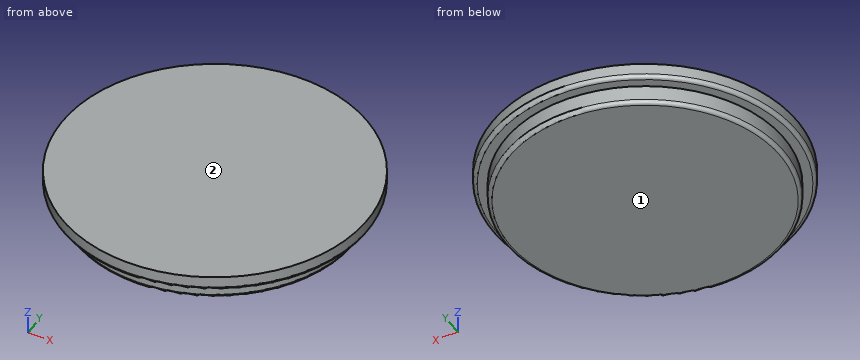
```python
from build123d import *

# Parameters (mm, degrees)
F0_R     = 18.75
F1_DEPTH = 2.5
F2_R     = 0.5
F3_R     = 20.5
F4_DEPTH = 2
F5_R     = 0.5


with BuildPart() as f1:
    # F0 (on Top) → F1 (new body)
    with BuildSketch(Plane.XY):
        Circle(F0_R)
    extrude(amount=F1_DEPTH)

    # F2
    f2_edges = [f1.edges().sort_by_distance(p)[0] for p in [
        (-18.75, 0, 0),
    ]]
    fillet(f2_edges, radius=F2_R)

    # F3 (on face) → F4 (join)
    with BuildSketch(Plane.XY.offset(2.5)):
        Circle(F3_R)
    extrude(amount=F4_DEPTH)

    # F5
    f5_edges = [f1.edges().sort_by_distance(p)[0] for p in [
        (-20.5, 0, 2.5),
    ]]
    fillet(f5_edges, radius=F5_R)


solid = f1.part
```
Verification items for the finished model (mm, model axes). Face numbers are marked on the shaded views. Coordinates: 2 decimals unless noted, no trailing zeros. Loops run counter-clockwise (first coordinate to the right, second up) from the corner with the lowest first, then second, coordinate; pieces in that order, holes last. Notation, with made-up numbers: (79.5, 72) - (136.5, 72) arc R13 cw to (136.5, 92) - close; hole circle Ø5 at (78.25, 55). An arc over 180 degrees is marked (long way). Answer as a JSON object with one key per item and string values.
(1) Mould release check, pull along Z, two halves, no side actions. Record for the marked faces 1 and 2: pulls with the +Z half, pulls with the -Z half, needs draft (parallel to the pull), parting line crosses it, or undercut.
Response:
{"face 1": "pulls with the -Z half", "face 2": "pulls with the +Z half"}
(2) Go/stop test with flat-tipped pins: pin 1 Ø1 at (x, z) = (-10.5, 1.5) entering from -Y; pin 2 Ø1 at (x, z) = (-6, 4) entering from +Y; pin 3 Ø1.5 at (y, z) = (7, 2) entering from -X. Record where each tip stops, or that it passes through.
Response:
{"pin 1": "stops at y = -15.86", "pin 2": "stops at y = 19.75", "pin 3": "stops at x = -19.26"}
(3) Scan lines: line 1 along Z through (x, y) = (-11, 15.5); line 2 along X through (y, z) = (-4, 3.55); line 3 along Y through (x, z) = (4.5, 1.55). Record each from-to range of solid material in increasing order.
Response:
{"line 1": "z = 2.5 to 4.5", "line 2": "x = -20.11 to 20.11", "line 3": "y = -18.2 to 18.2"}
(4) Cross-section at C-C, the plane z = 1.6. Record the boundary of the cut face in (x, y).
Response:
{"outline": "circle Ø37.5 at (0, 0)"}
(5) Cross-section at D-D, the plane z = 3.85. Record the boundary of the cut face in (x, y).
Response:
{"outline": "circle Ø41 at (0, 0)"}
(6) Cross-section at A-A, the plane y = 0. Record the boundary of the cut face in (x, z), then the cut area to 3 significant figures.
Response:
{"outline": "(-20.5, 3) arc R0.5 ccw to (-20, 2.5) - (-18.75, 2.5) - (-18.75, 0.5) arc R0.5 ccw to (-18.25, 0) - (18.25, 0) arc R0.5 ccw to (18.75, 0.5) - (18.75, 2.5) - (20, 2.5) arc R0.5 ccw to (20.5, 3) - (20.5, 4.5) - (-20.5, 4.5) - close", "area": "176 mm²"}
